Check sheet for the modelled part. Datum: model origin and axes. Units: mm. Face numbers are marked on the shaded views. A direction names the side the tool comes from. Round coordinates to 2 decimals unless told otherwise and drop trailing zeros. Loops run counter-clockwise (first coordinate to the right, second up) from the corner with the lowest first, then second, coordinate; pieces in that order, holes last. Notation, with made-up numbers: (75.5, -21.5) -> (100.5, -21.5) arc R34 ccw to (100.5, 17.5) -> close; hole circle Ø11 at (43, -0.75). An arc over 180 degrees is marked (long way). Use one line per item in the form item = value. Start each with the question number.
(1) Set-up check for the marked faces 1, 2 and 3: record each of +Z, -Z, +X, -X, +Y, -Y from which the full face is reachable in a straight line by a thin tool's end or side.
(2) Sectioned sample at A-A (x = -21.5). Record the cut outline in (y, z), and give its area (3 significant figures).
(3) Material ranges on probe 1 along Z at (x, y) = (-58, 68); probe 2 along X at (y, z) = (24.5, 11); probe 3 along Y at (x, z) = (-17.5, 6.5), recorded low to high. Write a range as [from, to].
(4) Go/stop test with flat-tipped pins: pin 1 (1.5 mm diameter, centred on x = -66, y = -1, fed in from +Z); pin 2 (1.5 mm diameter, centred on x = -61.5, y = 67, fed in from -Z); pin 3 (3.5 mm diameter, centred on x = -41.5, z = 10.5, fed in from -Y); pin 4 (2.5 mm diameter, centred on y = -1.5, z = 1.5, fed in from +X). Record where each tip stops, or that it passes through.
(5) Sectioned sample at B-B (z = 26.5). Record the cut outline in (x, y).
(6) Sectioned sample at D-D (z = 59). Record the cut outline in (x, y).
(7) Sectioned sample at C-C (y = 15.5). Record the cut outline in (x, z), and give its area (3 significant figures).
from build123d import *

# Parameters (mm, degrees)
BASE_FLANGE1_DEPTH           = 70
EDGE_FLANGE1_STRIP_W         = 16
EDGE_FLANGE1_STRIP_H         = 3
EDGE_FLANGE1_STRIP_CUT_DEPTH = 70
EDGE_FLANGE1_DEPTH           = 70
EDGE_FLANGE2_STRIP_W         = 16
EDGE_FLANGE2_STRIP_H         = 3
EDGE_FLANGE2_STRIP_CUT_DEPTH = 70
EDGE_FLANGE2_DEPTH           = 70
SKETCH19_W                   = 15
SKETCH19_H                   = 6
BOSS_EXTRUDE1_DEPTH          = 3
SKETCH20_W                   = 15
SKETCH20_H                   = 6
BOSS_EXTRUDE2_DEPTH          = 3
CUT_EXTRUDE6_DEPTH           = 3
EDGE_FLANGE8_STRIP_W         = 14
EDGE_FLANGE8_STRIP_H         = 3
EDGE_FLANGE8_STRIP_CUT_DEPTH = 30
EDGE_FLANGE8_DEPTH           = 30
SKETCH71_R                   = 2.1
CUT_EXTRUDE7_DEPTH           = 3
CUT_EXTRUDE8_DEPTH           = 3
EDGE_FLANGE9_STRIP_W         = 14
EDGE_FLANGE9_STRIP_H         = 3
EDGE_FLANGE9_STRIP_CUT_DEPTH = 30
EDGE_FLANGE9_DEPTH           = 30
SKETCH77_R                   = 2.1
CUT_EXTRUDE9_DEPTH           = 3
FILLET1_R                    = 1
FILLET2_R                    = 3


# Sheet-metal steps are written as plain solids
with BuildPart() as part:
    # Sketch1 → Base-Flange1 (new body)
    with BuildSketch(Plane(origin=(0, 0, 0), x_dir=(1, 0, 0), z_dir=(0, 1, 0))):
        with BuildLine():
            Line((0, 0), (-58, 0))
            ThreePointArc((-58, 0), (-65.071067812, -2.928932188), (-68, -10))
            Line((-68, -10), (-68, -68))
            Line((-68, -68), (-65, -68))
            Line((-65, -68), (-65, -10))
            ThreePointArc((-65, -10), (-62.949747468, -5.050252532), (-58, -3))
            Line((-58, -3), (0, -3))
            Line((0, -3), (0, 0))
        make_face()
    extrude(amount=BASE_FLANGE1_DEPTH)

    # Edge-Flange1 strip (across the edge) → Edge-Flange1 strip cut (cut)
    with BuildSketch(Plane(origin=(0, 0, 3), x_dir=(-1, 0, 0), z_dir=(0, 1, 0))):
        with Locations((-3, -1.5)):
            Rectangle(EDGE_FLANGE1_STRIP_W, EDGE_FLANGE1_STRIP_H)
    extrude(amount=EDGE_FLANGE1_STRIP_CUT_DEPTH, mode=Mode.SUBTRACT)

    # Edge-Flange1 section (across the edge) → Edge-Flange1 (add)
    with BuildSketch(Plane(origin=(0, 0, 3), x_dir=(-1, 0, 0), z_dir=(0, 1, 0))):
        with BuildLine():
            Line((0, 2), (0, 12))
            Line((0, 12), (3, 12))
            Line((3, 12), (3, 2))
            ThreePointArc((3, 2), (3.585786438, 0.585786438), (5, 0))
            Line((5, 0), (5, -3))
            ThreePointArc((5, -3), (1.464466094, -1.535533906), (0, 2))
        make_face()
    extrude(amount=EDGE_FLANGE1_DEPTH)

    # Edge-Flange2 strip (across the edge) → Edge-Flange2 strip cut (cut)
    with BuildSketch(Plane(origin=(-65, 70, 68), x_dir=(0, 0, -1), z_dir=(0, -1, 0))):
        with Locations((-3, -1.5)):
            Rectangle(EDGE_FLANGE2_STRIP_W, EDGE_FLANGE2_STRIP_H)
    extrude(amount=EDGE_FLANGE2_STRIP_CUT_DEPTH, mode=Mode.SUBTRACT)

    # Edge-Flange2 section (across the edge) → Edge-Flange2 (add)
    with BuildSketch(Plane(origin=(-65, 70, 68), x_dir=(0, 0, -1), z_dir=(0, -1, 0))):
        with BuildLine():
            Line((0, 2), (0, 12))
            Line((0, 12), (3, 12))
            Line((3, 12), (3, 2))
            ThreePointArc((3, 2), (3.585786438, 0.585786438), (5, 0))
            Line((5, 0), (5, -3))
            ThreePointArc((5, -3), (1.464466094, -1.535533906), (0, 2))
        make_face()
    extrude(amount=EDGE_FLANGE2_DEPTH)

    # Sketch19 → Boss-Extrude1 (add)
    with BuildSketch(Plane.XY.offset(3)):
        with Locations((-31.5, 0)):
            Rectangle(SKETCH19_W, SKETCH19_H)
    extrude(amount=-BOSS_EXTRUDE1_DEPTH)

    # Sketch20 → Boss-Extrude2 (add)
    with BuildSketch(Plane(origin=(-65, 0, 0), x_dir=(0, 0, -1), z_dir=(1, 0, 0))):
        with Locations((-36.5, 0)):
            Rectangle(SKETCH20_W, SKETCH20_H)
    extrude(amount=-BOSS_EXTRUDE2_DEPTH)

    # Sketch63 → Cut-Extrude6 (cut)
    with BuildSketch(Plane(origin=(-65, 0, 0), x_dir=(0, 0, -1), z_dir=(1, 0, 0))):
        Polygon((-51.5, 64), (-51.5, 67), (-51.5, 70), (-53.5, 70), (-53.5, 64), align=None)
        Polygon((-21.5, 70), (-21.5, 67), (-21.5, 64), (-19.5, 64), (-19.5, 70), align=None)
    extrude(amount=-CUT_EXTRUDE6_DEPTH, mode=Mode.SUBTRACT)

    # Edge-Flange8 strip (across the edge) → Edge-Flange8 strip cut (cut)
    with BuildSketch(Plane(origin=(-65, 70, 21.5), x_dir=(0, -1, 0), z_dir=(0, 0, 1))):
        with Locations((-3, -1.5)):
            Rectangle(EDGE_FLANGE8_STRIP_W, EDGE_FLANGE8_STRIP_H)
    extrude(amount=EDGE_FLANGE8_STRIP_CUT_DEPTH, mode=Mode.SUBTRACT)

    # Edge-Flange8 section (across the edge) → Edge-Flange8 (add)
    with BuildSketch(Plane(origin=(-65, 70, 21.5), x_dir=(0, -1, 0), z_dir=(0, 0, 1))):
        with BuildLine():
            Line((0, 1), (0, 12))
            Line((0, 12), (3, 12))
            Line((3, 12), (3, 1))
            ThreePointArc((3, 1), (3.292893219, 0.292893219), (4, 0))
            Line((4, 0), (4, -3))
            ThreePointArc((4, -3), (1.171572875, -1.828427125), (0, 1))
        make_face()
    extrude(amount=EDGE_FLANGE8_DEPTH)

    # Sketch71 → Cut-Extrude7 (cut)
    with BuildSketch(Plane(origin=(0, 70, 0), x_dir=(1, 0, 0), z_dir=(0, 1, 0))):
        with Locations(Location((-58.5, -26.5, 0), (0, 0, 180))):
            Circle(SKETCH71_R)
        with Locations(Location((-58.5, -46.5, 0), (0, 0, 180))):
            Circle(SKETCH71_R)
    extrude(amount=-CUT_EXTRUDE7_DEPTH, mode=Mode.SUBTRACT)

    # Sketch72 → Cut-Extrude8 (cut)
    with BuildSketch(Plane.XY.offset(3)):
        Polygon((-46.5, 66.882619945), (-46.5, 70), (-48.5, 70), (-48.5, 64), (-46.5, 64), align=None)
        Polygon((-14.5, 70), (-16.5, 70), (-16.5, 66.882619945), (-16.5, 64), (-14.5, 64), align=None)
    extrude(amount=-CUT_EXTRUDE8_DEPTH, mode=Mode.SUBTRACT)

    # Edge-Flange9 strip (across the edge) → Edge-Flange9 strip cut (cut)
    with BuildSketch(Plane(origin=(-16.5, 70, 3), x_dir=(0, -1, 0), z_dir=(-1, 0, 0))):
        with Locations((-3, -1.5)):
            Rectangle(EDGE_FLANGE9_STRIP_W, EDGE_FLANGE9_STRIP_H)
    extrude(amount=EDGE_FLANGE9_STRIP_CUT_DEPTH, mode=Mode.SUBTRACT)

    # Edge-Flange9 section (across the edge) → Edge-Flange9 (add)
    with BuildSketch(Plane(origin=(-16.5, 70, 3), x_dir=(0, -1, 0), z_dir=(-1, 0, 0))):
        with BuildLine():
            Line((0, 1), (0, 12))
            Line((0, 12), (3, 12))
            Line((3, 12), (3, 1))
            ThreePointArc((3, 1), (3.292893219, 0.292893219), (4, 0))
            Line((4, 0), (4, -3))
            ThreePointArc((4, -3), (1.171572875, -1.828427125), (0, 1))
        make_face()
    extrude(amount=EDGE_FLANGE9_DEPTH)

    # Sketch77 → Cut-Extrude9 (cut)
    with BuildSketch(Plane(origin=(0, 70, 0), x_dir=(1, 0, 0), z_dir=(0, 1, 0))):
        with Locations(Location((-41.5, -10.5, 0), (0, 0, 270))):
            Circle(SKETCH77_R)
        with Locations(Location((-21.5, -10.5, 0), (0, 0, 270))):
            Circle(SKETCH77_R)
    extrude(amount=-CUT_EXTRUDE9_DEPTH, mode=Mode.SUBTRACT)

    # Fillet1
    fillet1_edges = [part.edges().sort_by_distance(p)[0] for p in [
        (-66.5, 70, 53.5),
        (-66.5, 64, 53.5),
        (-66.5, 64, 51.5),
        (-66.5, 64, 21.5),
        (-66.5, 64, 19.5),
        (-66.5, 70, 19.5),
        (-14.5, 70, 1.5),
        (-48.5, 70, 1.5),
        (-14.5, 64, 1.5),
        (-16.5, 64, 1.5),
        (-46.5, 64, 1.5),
        (-48.5, 64, 1.5),
    ]]
    fillet(fillet1_edges, radius=FILLET1_R - 0.0001)  # a hair under: the kernel refuses the full size

    # Fillet2
    fillet2_edges = [part.edges().sort_by_distance(p)[0] for p in [
        (-1.5, 70, 15),
        (-1.5, 0, 15),
        (-53, 0, 66.5),
        (-53, 70, 66.5),
        (-53, 68.5, 21.5),
        (-53, 68.5, 51.5),
        (-16.5, 68.5, 15),
        (-46.5, 68.5, 15),
    ]]
    fillet(fillet2_edges, radius=FILLET2_R)


solid = part.part
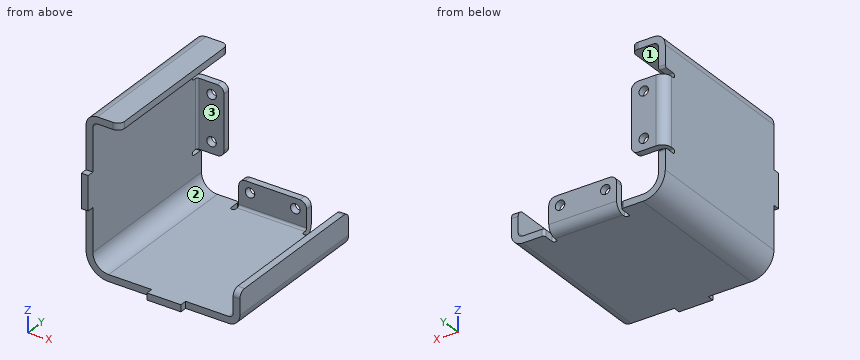
Checks:
q1.face_1 = +X, +Y, -Y
q1.face_2 = +Y, -Y
q1.face_3 = +X, -Y
q2.outline = (0, 0) -> (66, 0) arc R4 ccw to (70, 4) -> (70, 8.4) -> (67, 8.4) -> (67, 4) arc R1 cw to (66, 3) -> (0, 3) -> close; (67, 12.6) -> (70, 12.6) -> (70, 15) -> (67, 15) -> close
q2.area = 230 mm2
q3.probe_1 = [0, 3], [21.5, 24.46], [28.54, 44.46], [48.54, 51.5], [65, 68]
q3.probe_2 = [-68, -65], [-3, 0]
q3.probe_3 = [67, 70]
q4.pin_1 = 44
q4.pin_2 = 0.39
q4.pin_3 = through
q4.pin_4 = -24
q5.outline = (-68, 0) -> (-65, 0) -> (-65, 66) arc R1 cw to (-64, 67) -> (-60.6, 67) -> (-60.6, 70) -> (-64, 70) arc R4 ccw to (-68, 66) -> close; (-56.4, 67) -> (-53, 67) -> (-53, 70) -> (-56.4, 70) -> close
q6.outline = (-68, 0) -> (-65, 0) -> (-65, 70) -> (-68, 70) -> close
q7.outline = (-68, 10) arc R10 ccw to (-58, 0) -> (-5, 0) arc R5 ccw to (0, 5) -> (0, 15) -> (-3, 15) -> (-3, 5) arc R2 cw to (-5, 3) -> (-58, 3) arc R7 cw to (-65, 10) -> (-65, 63) arc R2 cw to (-63, 65) -> (-53, 65) -> (-53, 68) -> (-63, 68) arc R5 ccw to (-68, 63) -> close
q7.area = 451 mm2
